Check sheet for the drawn part. Datum: minimum x, y, z corner. Units: mm. Round coordinates to 2 decimals unless told otherwise and drop trailing zeros. Loops run counter-clockwise (first coordinate to the right, second up) from the corner with the lowest first, then second, coordinate; pieces in that order, holes last.
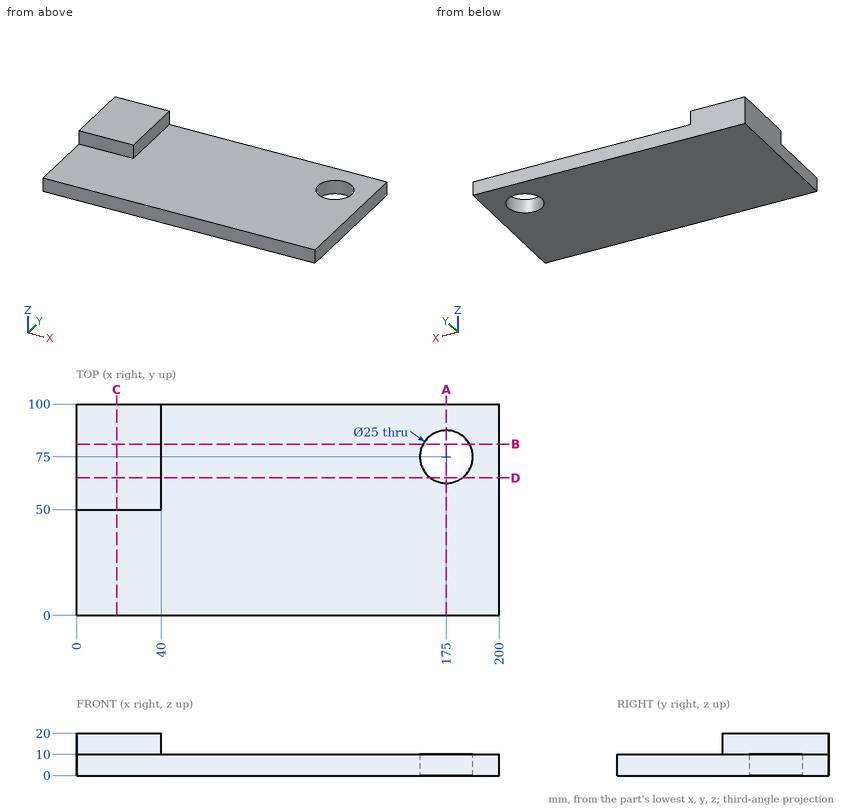
1) Sectioned sample at B-B, the plane y = 81. Record the cut outline in (x, z).
Report:
outline: (0, 0) - (164.03, 0) - (164.03, 10) - (40, 10) - (40, 20) - (0, 20) - close; (185.97, 0) - (200, 0) - (200, 10) - (185.97, 10) - close
2) Sectioned sample at C-C, the plane x = 19. Record the cut outline in (y, z).
Report:
outline: (0, 0) - (100, 0) - (100, 20) - (50, 20) - (50, 10) - (0, 10) - close
3) Sectioned sample at A-A, the plane x = 175. Record the cut outline in (y, z), then the cut area to 3 significant figures.
Report:
outline: (0, 0) - (62.5, 0) - (62.5, 10) - (0, 10) - close; (87.5, 0) - (100, 0) - (100, 10) - (87.5, 10) - close
area: 750 mm2
4) Scan lines: line 1 along Y through (x, z) = (175, 3); line 2 along X through (y, z) = (78, 15.75); line 3 along Z through (x, y) = (158.5, 22.5). Record each from-to range of solid material in increasing order.
Report:
line 1: y = 0 to 62.5, 87.5 to 100
line 2: x = 0 to 40
line 3: z = 0 to 10
5) Sectioned sample at D-D, the plane y = 65. Record the cut outline in (x, z).
Report:
outline: (0, 0) - (167.5, 0) - (167.5, 10) - (40, 10) - (40, 20) - (0, 20) - close; (182.5, 0) - (200, 0) - (200, 10) - (182.5, 10) - close
6) Gauge pin test, flat ends, axial feed: pin 1 (5 mm diameter, centred on x = 22.5, z = 13, fed in from -Y); pin 2 (3 mm diameter, centred on x = 82.5, y = 18.5, fed in from +Z). Record the tip position at first contact, or that the pin passes through.
Report:
pin 1: stops at y = 50
pin 2: stops at z = 10
